```python
from build123d import *

# Parameters (mm, degrees)
SKETCH1_W           = 327.074
SKETCH1_H           = 26.4
SKETCH1_W_2         = 313.074
SKETCH1_H_2         = 12.4
BOSS_EXTRUDE1_DEPTH = 20
SKETCH2_W           = 327.074
SKETCH2_H           = 242.4
BOSS_EXTRUDE2_DEPTH = 3.175
SKETCH3_W           = 327.074
SKETCH3_H           = 216
BOSS_EXTRUDE3_DEPTH = 134.85
CUT_EXTRUDE1_REACH  = 400.252
CUT_EXTRUDE2_REACH  = 398.452
SKETCH5_W           = 307.074
SKETCH5_H           = 118.025


with BuildPart() as part:
    # Sketch1 → Boss-Extrude1 (new body)
    with BuildSketch(Plane(origin=(0, 0, 0), x_dir=(1, 0, 0), z_dir=(0, 1, 0))):
        with Locations((-119.715833623, 46.325831873)):
            Rectangle(SKETCH1_W, SKETCH1_H)
        with Locations((-119.715833623, 46.325831873)):
            Rectangle(SKETCH1_W_2, SKETCH1_H_2, mode=Mode.SUBTRACT)
    extrude(amount=BOSS_EXTRUDE1_DEPTH)

    # Sketch2 → Boss-Extrude2 (add)
    with BuildSketch(Plane.XZ):
        with Locations((-119.715833623, 61.674168127)):
            Rectangle(SKETCH2_W, SKETCH2_H)
    extrude(amount=BOSS_EXTRUDE2_DEPTH)

    # Sketch3 → Boss-Extrude3 (add)
    with BuildSketch(Plane(origin=(0, 0, 0), x_dir=(1, 0, 0), z_dir=(0, 1, 0))):
        with Locations((-119.715833623, -74.874168127)):
            Rectangle(SKETCH3_W, SKETCH3_H)
    extrude(amount=BOSS_EXTRUDE3_DEPTH)

    # Sketch4 → Cut-Extrude1 (cut, up to next)
    with BuildSketch(Plane.ZY.offset(283.252833623), mode=Mode.PRIVATE) as cut_extrude1_sk1:
        Polygon((-23.125831873, 10), (-23.125831873, 6.825), (172.874168127, 6.825), (172.874168127, 124.85), (-23.125831873, 124.85), align=None)
    cut_extrude1_tool1 = extrude(cut_extrude1_sk1.sketch, amount=-CUT_EXTRUDE1_REACH, mode=Mode.PRIVATE) & part.part
    add(cut_extrude1_tool1.solids().sort_by_distance((-283.252834, 65.8375, 74.874168))[0], mode=Mode.SUBTRACT)

    # Cut-Extrude2: up to this face of the body (flat: up to its plane)
    cut_extrude2_end = Plane(part.part.faces().sort_by_distance((-119.715833623, 77.425, -33.125831873))[0])
    # Sketch5 → Cut-Extrude2 (cut, up to the picked face)
    with BuildSketch(Plane.XY.offset(182.874168127), mode=Mode.PRIVATE) as cut_extrude2_sk1:
        with Locations((-119.715833623, 65.8375)):
            Rectangle(SKETCH5_W, SKETCH5_H)
    cut_extrude2_tool1 = split(extrude(cut_extrude2_sk1.sketch, amount=-CUT_EXTRUDE2_REACH, mode=Mode.PRIVATE), bisect_by=cut_extrude2_end, keep=Keep.BOTH, mode=Mode.PRIVATE)
    add(cut_extrude2_tool1.solids().sort_by(Axis((-119.715834, 65.8375, 182.874168), (0, 0, -1)))[0], mode=Mode.SUBTRACT)


solid = part.part
```
Source: CAD feature listing. Evaluate the final solid. Frame: model axes, mm. A direction names the side the tool comes from. Give positions to 0.01 mm unless a question says otherwise; leave off trailing zeros. Order: outer loops, then holes, each group sorted by start corner. A loop starts at its lowest first (then second) coordinate and runs counter-clockwise, first axis right, second up.
(1) Section query B-B (z = 105). Return the cut outline in (x, y) (3 decimals).
(2) Section query C-C (y = 38). Return the cut outline in (x, z).
(3) Section query A-A (x = -165). Return the cut outline in (y, z) (3 decimals).
(4) Material intervals for line 1 along Z through (x, y) = (-119, 18); line 2 along Y through (x, z) = (-270, -28) (3 decimals); line 3 along X through (y, z) = (8.5, -45), sorted ascending.
(5) Pull-direction query (X, two-part tool) for faces 5 (the face through (-273.253, 65, -28)), 6 (the face through (43.821, 4, 62)), 7 (the face through (-278, 67, -23.126)); classes: +X half, -X half, draft (parallel to the pull), parting line (faces both ways), or undercut.
(6) Access query for faces 1 (the face through (-122, 13, -33.126)), 2 (the face through (39, 67, -23.126)), 3 (the face through (-120, 128, -33.126)), 4 (the face through (-122, 10, -40.126)). Directions: +Z, -Z, +X, -X, +Y, -Y. A direction counts if a zero-diameter tool reaches every point of the face in a straight line with its end or side. Return the directions, or none.
(7) Contact query for flat-ended pins moving along their axis: P1, Ø8, axis at x = -191.5, y = 120.5, coming from the -Z side; P2, Ø21, axis at x = -193.5, z = -42.5, coming from the +Y side; P3, Ø3.5, axis at x = -103, z = -48.5, coming from the +Y side; P4, Ø11, axis at x = 38.5, y = 42, coming from the -Z side. Output: stop coordinate, or through.
Outcome:
1. outline: (-283.253, -3.175) - (43.821, -3.175) - (43.821, 6.825) - (-283.253, 6.825) - close; (-283.253, 124.85) - (43.821, 124.85) - (43.821, 134.85) - (-283.253, 134.85) - close
2. outline: (-283.25, -33.13) - (-273.25, -33.13) - (-273.25, -23.13) - (-283.25, -23.13) - close; (-283.25, 172.87) - (-273.25, 172.87) - (-273.25, 182.87) - (-283.25, 182.87) - close; (33.82, -33.13) - (43.82, -33.13) - (43.82, -23.13) - (33.82, -23.13) - close; (33.82, 172.87) - (43.82, 172.87) - (43.82, 182.87) - (33.82, 182.87) - close
3. outline: (-3.175, -59.526) - (20, -59.526) - (20, -52.526) - (0, -52.526) - (0, -40.126) - (20, -40.126) - (20, -33.126) - (6.825, -33.126) - (6.825, 182.874) - (-3.175, 182.874) - close; (124.85, -33.126) - (134.85, -33.126) - (134.85, 182.874) - (124.85, 182.874) - close
4. line 1: z = -59.53 to -52.53, -40.13 to -33.13
4. line 2: y = -3.175 to 6.825, 124.85 to 134.85
4. line 3: x = -283.25 to -276.25, 36.82 to 43.82
5. face 5: undercut
5. face 6: +X half
5. face 7: draft
6. face 1: +Z
6. face 2: +X, -X
6. face 3: -Z, +X, -X, +Y
6. face 4: +Y
7. P1: passes through
7. P2: stops at y = 134.85
7. P3: stops at y = 0
7. P4: stops at z = -33.13
